```python
from build123d import *

# Parameters (mm, degrees)
SKETCH_R     = 2
PAD_DEPTH    = 5
CHAMFER_SIZE = 2


with BuildPart() as part:
    # Sketch → Pad (new body)
    with BuildSketch(Plane.XY):
        with BuildLine():
            Line((-60, 30), (-60, -30))
            ThreePointArc((-60, -30), (-58.535534, -33.535534), (-55, -35))
            Line((-55, -35), (55, -35))
            ThreePointArc((55, -35), (58.535534, -33.535534), (60, -30))
            Line((60, -30), (60, 30))
            ThreePointArc((60, 30), (58.535534, 33.535534), (55, 35))
            Line((55, 35), (-55, 35))
            ThreePointArc((-55, 35), (-58.535534, 33.535534), (-60, 30))
        make_face()
        with Locations((-45, 0)):
            Circle(SKETCH_R, mode=Mode.SUBTRACT)
        with Locations((45, 0)):
            Circle(SKETCH_R, mode=Mode.SUBTRACT)
    extrude(amount=PAD_DEPTH)

    # Chamfer
    chamfer_edges = [part.edges().sort_by_distance(p)[0] for p in [
        (-60, 0, 5),
        (-58.535534, -33.535534, 5),
        (0, -35, 5),
        (58.535534, -33.535534, 5),
        (60, 0, 5),
        (58.535534, 33.535534, 5),
        (0, 35, 5),
        (-58.535534, 33.535534, 5),
        (43, 0, 5),
        (-47, 0, 5),
    ]]
    chamfer(chamfer_edges, length=CHAMFER_SIZE)


solid = part.part
```
Input: part model. Units: mm. Frame: model coordinates. Coordinates: 2 decimals unless noted, no trailing zeros. Write each loop counter-clockwise with the first axis right and the second up, starting at its lowest first coordinate (ties: lowest second). Pieces come first, ordered by that corner, then holes. Notation, with made-up numbers: (78.5, 45) -> (132.5, 45) arc R13 ccw to (132.5, 56) -> close; hole circle Ø11 at (26.5, 73). An arc over 180 degrees is marked (long way). Write each question's results on one line, items separated by ' | '.
Item 1: Pin query (flat end, axial travel): pin 1 Ø8 at (x, y) = (-20, 12.5) entering from -Z. Return the tip coordinate at first contact, or that it passes through.
Conclusion:
pin 1: stops at z = 0
Item 2: Mould query, pull axis Y, two halves, no side actions, for faces 1 (the conical face through (57.69, 32.63, 4.24)), 2 (the cylindrical face through (-47, 0, 1)), 3 (the conical face through (-57.69, -32.63, 4.24)). Classes: +Y half, -Y half, draft (parallel to the pull), parting line (faces both ways), or undercut.
Conclusion:
face 1: +Y half | face 2: undercut | face 3: -Y half
Item 3: Section query B-B on y = 0. Return loops of the section in (x, z), plus the area to 3 significant figures.
Conclusion:
outline: (-60, 0) -> (-47, 0) -> (-47, 3) -> (-49, 5) -> (-58, 5) -> (-60, 3) -> close; (-43, 0) -> (43, 0) -> (43, 3) -> (41, 5) -> (-41, 5) -> (-43, 3) -> close; (47, 0) -> (60, 0) -> (60, 3) -> (58, 5) -> (49, 5) -> (47, 3) -> close | area: 548 mm^2
Item 4: Material intervals for probe 1 along Y at (x, z) = (45, 1.25); probe 2 along X at (y, z) = (-1, 1.45); probe 3 along X at (y, z) = (22.5, 3.55), sorted ascending.
Conclusion:
probe 1: y = -35 to -2, 2 to 35 | probe 2: x = -60 to -46.73, -43.27 to 43.27, 46.73 to 60 | probe 3: x = -59.45 to 59.45
Item 5: Section query A-A on x = -45. Return loops of the section in (y, z).
Conclusion:
outline: (-35, 0) -> (-2, 0) -> (-2, 3) -> (-4, 5) -> (-33, 5) -> (-35, 3) -> close; (2, 0) -> (35, 0) -> (35, 3) -> (33, 5) -> (4, 5) -> (2, 3) -> close
